Geometry check sheet. Reference: the model listing, model coordinates, mm. Face numbers are marked on the shaded views. A direction names the side the tool comes from. Round coordinates to 2 decimals unless told otherwise and drop trailing zeros. Order: outer loops, then holes, each group sorted by start corner. A loop starts at its lowest first (then second) coordinate and runs counter-clockwise, first axis right, second up.
(1) Thickness scan on L1, parallel to Y at x = 0, z = 23; L2, parallel to Z at x = -1.5, y = -0.5; L3, parallel to X at y = -7, z = 42.5 (1 decimal). Record the ranges inside material, lowest first.
(2) Cross-section at A-A on y = 0. Enter the section's corners in (x, z), and give its area (3 significant figures).
(3) Gauge pin test, flat ends, axial feed: P1, Ø8, axis at x = 4, y = 10.5, coming from the +Z side; P2, Ø2, axis at x = -15, y = -5.5, coming from the +Z side; P3, Ø5, axis at x = -15.5, z = 40, coming from the +Y side; P4, Ø3, axis at x = -3, y = -5.5, coming from the -Z side. Record the tip position at first contact, or that the pin passes through.
(4) Set-up check for the marked faces 3 and 4: record each of +Z, -Z, +X, -X, +Y, -Y from which the full face is reachable in a straight line by a thin tool's end or side.
(5) Cross-section at C-C on z = 25. Enter the section's corners in (x, y), and give its area (3 significant figures).
(6) Cross-section at D-D on z = -28. Enter the section's corners in (x, y).
(7) Draft check along X on the marked faces 1 and 2. Enter one of: pulls with the +X half, pulls with the -X half, needs draft (parallel to the pull), parting line crosses it, or undercut.
Autodesk Inventor part; units mm, degrees
ref_plane "YZ Plane" through (0, 0, 0) normal (1, 0, 0) x (0, 1, 0)
ref_plane "XZ Plane" through (0, 0, 0) normal (0, 1, 0) x (-1, 0, 0)
ref_plane "XY Plane" through (0, 0, 0) normal (0, 0, 1) x (1, 0, 0)
sketch "スケッチ1" plane through (0, 0, 0) normal (0, 1, 0) x (-1, 0, 0)
  line L0 (0, 0) -> (20, 0) construction
  line L1 (20, 0) -> (20, 50)
  line L2 (20, 50) -> (0, 50)
  line L3 (20, 0) -> (0, 0)
  line L4 (0, 50) -> (0, 0)
  dimension "d4" = 50
  dimension "d12" = 20
revolve "回転1" add sketch "スケッチ1" angle 360 about axis through (0, 0, 50) along (0, 0, -1)
shell "シェル1" thickness 4 removed faces 1 at (-2.364, 6.2334, 50)
sketch "スケッチ2" plane through (0, 0, 0) normal (0, 1, 0) x (-1, 0, 0)
  line L0 (-20, 0) -> (20, 0)
  line L1 (0, -17.2687) -> (0, 0)
  line L2 (0, 0) -> (20, 0)
  line L3 (0, -17.2687) -> (0, -37.2687)
  line L4 (0, -37.2687) -> (3, -37.2687)
  line L5 (3, -37.2687) -> (3, -15.5418)
  line L6 (20, 0) -> (3, -15.5418)
  dimension "d9" = 20
  dimension "d10" = 3
revolve "回転2" add sketch "スケッチ2" angle 360 about axis through (0, 0, -17.2687) along (0, 0, 1)
properties part number "promo1"
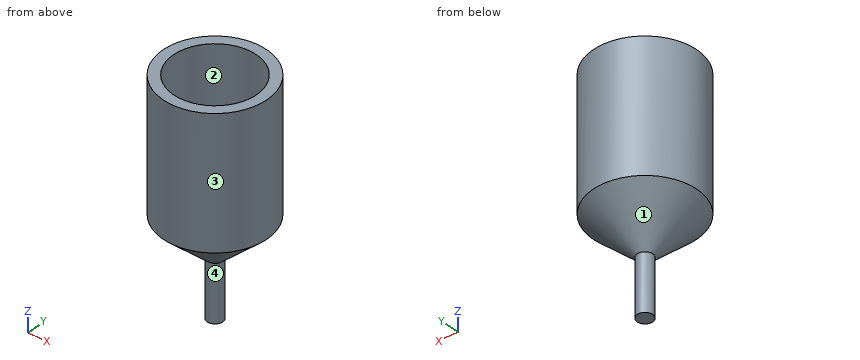
Found:
1. L1: y = -20 to -16, 16 to 20
1. L2: z = -37.27 to 4
1. L3: x = -18.7 to -14.4, 14.4 to 18.7
2. outline: (-20, 0) - (-3, -15.54) - (-3, -37.27) - (3, -37.27) - (3, -15.54) - (20, 0) - (20, 50) - (16, 50) - (16, 4) - (-16, 4) - (-16, 50) - (-20, 50) - close
2. area: 1,020 mm2
3. P1: stops at z = 4
3. P2: stops at z = 50
3. P3: stops at y = 15.2
3. P4: stops at z = -13.93
4. face 3: +Z, -Z
4. face 4: -Z
5. outline: circle Ø40 at (0, 0); hole circle Ø32 at (0, 0)
5. area: 452 mm2
6. outline: circle Ø6 at (0, 0)
7. face 1: parting line crosses it
7. face 2: undercut
